CAD build for the part. Positions are in the model's coordinates, mm. Round coordinates to 2 decimals unless told otherwise and drop trailing zeros. Return JSON: item names as keys, results as strings. Group by question number.
Q1. Probe line 1 along Y through (x, z) = (43.25, 7.1); line 2 along X through (y, z) = (80.5, 8.6) (3 decimals); line 3 along X through (y, z) = (83, 8.7) (3 decimals). List the from-to ranges inside material, lowest first.
Q2. Flat gauge pins, fed straight in: pin 1 (4 mm diameter, centred on x = 170.52, y = 9.4, fed in from +Z); pin 2 (0.9 mm diameter, centred on x = 58, z = 7.5, fed in from -Y); pin 3 (1 mm diameter, centred on x = 84.5, z = 8, fed in from -Y); pin 4 (0.9 mm diameter, centred on y = 83.5, z = 8, fed in from +X). Where does each tip first touch, or does it go through?
Q3. Cut at A-A (z = 7.6). Count the separate pieces of the cut face and the enclosed holes in it, then the cut area to 3 significant figures.
from build123d import *

# Parameters (mm, degrees)
PAD004_DEPTH    = 3
POCKET007_DEPTH = 5
SKETCH037_R     = 1.45
POCKET021_DEPTH = 9
FILLET002_R     = 1.5


with BuildPart() as part:
    # Sketch021 → Pad004 (new body)
    with BuildSketch(Plane.XY):
        with BuildLine():
            Line((85.725, 98.4875), (66.675, 98.4875))
            add(Edge.make_bspline(
                [(-8, 84.2), (39.625, 84.2), (39.625, 98.4875), (66.675, 98.4875)],
                knots=[0, 0, 0, 0, 1, 1, 1, 1], degree=3))
            Line((-8, 84.2), (-8, -8))
            add(Edge.make_bspline(
                [(39.625, -17.525), (39.625, -8), (20.575, -8), (-8, -8)],
                knots=[0, 0, 0, 0, 1, 1, 1, 1], degree=3))
            add(Edge.make_bspline(
                [(153.231854, -38.154949), (107.082107, -17.525), (76.2, -17.525), (39.625, -17.525)],
                knots=[0, 0, 0, 0, 1, 1, 1, 1], degree=3))
            Line((153.231854, -38.154949), (175.310198, 11.234895))
            add(Edge.make_bspline(
                [(150.875, 88.9625), (150.875, 42.8625), (150.875, 22.157965), (175.310198, 11.234895)],
                knots=[0, 0, 0, 0, 1, 1, 1, 1], degree=3))
            add(Edge.make_bspline(
                [(85.725, 98.4875), (104.775, 98.4875), (104.775, 88.9625), (150.875, 88.9625)],
                knots=[0, 0, 0, 0, 1, 1, 1, 1], degree=3))
        make_face()
    extrude(amount=PAD004_DEPTH)

    # Sketch023 → Pocket007 (cut)
    with BuildSketch(Plane(origin=(0, 0, 0), x_dir=(1, 0, 0), z_dir=(0, 0, -1))):
        Polygon((-0.75, 0.75), (-0.75, -76.95), (46.875, -76.95), (46.875, -86.475), (65.925, -86.475), (65.925, -91.2375), (86.475, -91.2375), (86.475, -86.475), (105.525, -86.475), (105.525, -81.7125), (143.625, -81.7125), (143.625, -17.457464), (165.732668, -7.574851), (149.57181, 28.577419), (131.568158, 20.529392), (102.96164, 14.448889), (103.848827, 10.275), (84.975, 10.275), (84.975, 5.5125), (67.425, 5.5125), (67.425, 10.275), (46.875, 10.275), (46.875, 0.75), align=None)
    extrude(amount=-POCKET007_DEPTH, mode=Mode.SUBTRACT)

    # Sketch037 → Pocket021 (cut)
    with BuildSketch(Plane.XY):
        with Locations((-4.375, -4.375)):
            Circle(SKETCH037_R)
        with Locations((-4.375, 80.575)):
            Circle(SKETCH037_R)
        with Locations((151.401832, -33.366184)):
            Circle(SKETCH037_R)
        with Locations((170.521433, 9.404873)):
            Circle(SKETCH037_R)
        with Locations((147.25, 85.3375)):
            Circle(SKETCH037_R)
        with Locations((43.25, -13.9)):
            Circle(SKETCH037_R)
        with Locations((57.15, 92.085)):
            Circle(SKETCH037_R)
        with Locations((95.25, 92.085)):
            Circle(SKETCH037_R)
        with Locations((95.25, -13.9)):
            Circle(SKETCH037_R)
    extrude(amount=POCKET021_DEPTH, mode=Mode.SUBTRACT)

    # Fillet002
    fillet002_edges = [part.edges().sort_by_distance(p)[0] for p in [
        (-8, -8, 1.5),
        (-8, 84.2, 1.5),
        (150.875, 88.9625, 1.5),
        (175.310198, 11.234895, 1.5),
        (153.231854, -38.154949, 1.5),
        (39.625, -17.525, 1.5),
    ]]
    fillet(fillet002_edges, radius=FILLET002_R)


with BuildPart() as part_1:
    # Body003 placement: moved
    add(part.part.moved(Location((0, 0, 6))))


solid = part_1.part
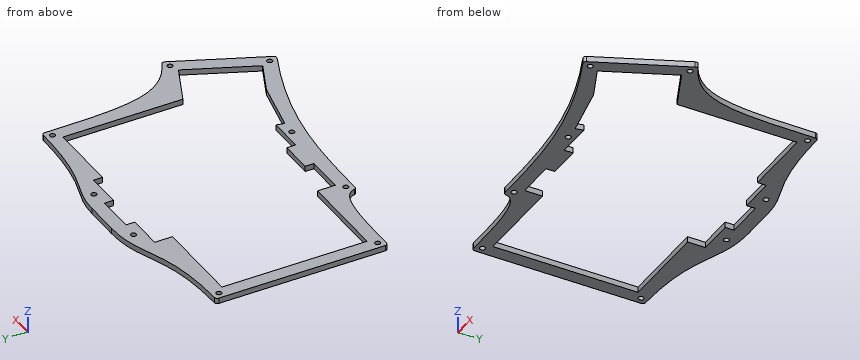
Solution:
{
 "1": {"line 1": "y = -17.53 to -15.35, -12.45 to -0.75, 76.95 to 93.78", "line 2": "x = -8 to -5.823, -2.927 to 46.875, 143.625 to 150.881", "line 3": "x = -7.971 to 46.875, 105.525 to 150.877"},
 "2": {"pin 1": "stops at z = 9", "pin 2": "stops at y = -17.64", "pin 3": "stops at y = -19.13", "pin 4": "stops at x = 150.88"},
 "3": {"separate pieces": "1", "enclosed holes": "10", "area": "4,640 mm²"}
}
